Can you work these out from the drawing? Everything is in mm from the part's minimum corner. A direction names the side the tool comes from. Round coordinates to 2 decimals unless told otherwise and drop trailing zeros. Loops run counter-clockwise (first coordinate to the right, second up) from the corner with the lowest first, then second, coordinate; pieces in that order, holes last. Notation, with made-up numbers: (71.25, -27.5) - (129.25, -27.5) arc R22 ccw to (129.25, 11.5) - close; hole circle Ø10 at (42, 18). An arc over 180 degrees is marked (long way). Return JSON: item names as keys, results as strings. Group by question number.
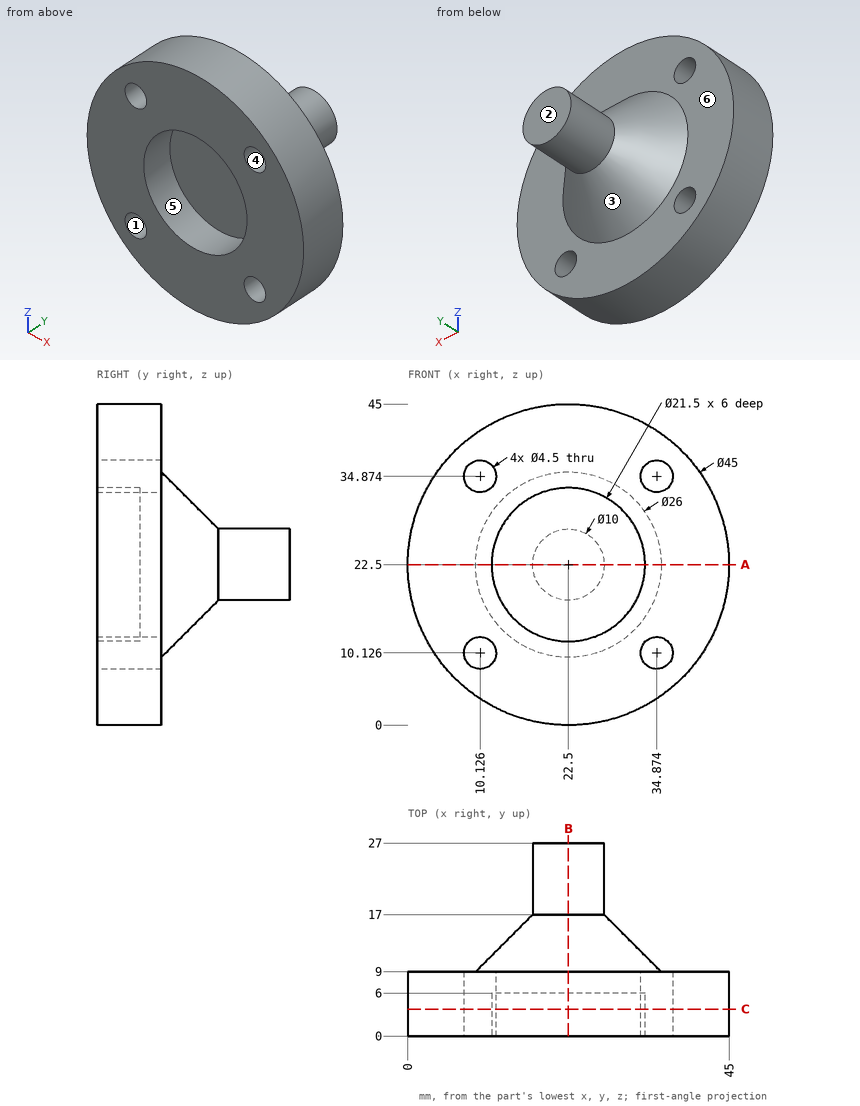
Q1. Imagine slicing it at A-A, the plane z = 22.5. List the corners of the cut face in (x, y) for me, and give its area (3 significant figures).
Q2. Will these pins go through, and if not, where does the flat tip stop? pin 1 Ø12 at (y, z) = (3.5, 39) entering from -X; pin 2 Ø3.5 at (x, z) = (34.87, 34.87) entering from +Y; pin 3 Ø11 at (x, z) = (22, 19.5) entering from -Y; pin 4 Ø5 at (x, z) = (34.87, 10.13) entering from -Y.
Q3. Imagine slicing it at C-C, the plane y = 3.75. Give the number of separate pieces and of enclosed holes in the cut face, and give its area (3 significant figures).
Q4. Imagine slicing it at B-B, the plane x = 22.5. List the corners of the cut face in (y, z) for me.
Q5. If we mould it in two halves opening along X, with no side actions, what happens to the marked faces 1, 2 and 3? For each: +X half, -X half, draft (parallel to the pull), parting line (faces both ways), or undercut.
Q6. For the marked faces 4, 5 and 6, which set-ups out of +Z, -Z, +X, -X, +Y, -Y let a thin tool reach every point of the face, with its end or its side?
Q7. Please list where these lines run through material, in increasing order: line 1 (Z direction, x = 36, y = 7.5) (1 decimal); line 2 (Z direction, x = 22.5, y = 4); line 3 (Z direction, x = 11, y = 1.5).
Output values:
{
 "1": {"outline": "(0, 0) - (11.75, 0) - (11.75, 6) - (33.25, 6) - (33.25, 0) - (45, 0) - (45, 9) - (35.5, 9) - (27.5, 17) - (27.5, 27) - (17.5, 27) - (17.5, 17) - (9.5, 9) - (0, 9) - close", "area": "520 mm^2"},
 "2": {"pin 1": "stops at x = 2.6", "pin 2": "passes through", "pin 3": "stops at y = 6", "pin 4": "stops at y = 0"},
 "3": {"separate pieces": "1", "enclosed holes": "5", "area": "1,160 mm^2"},
 "4": {"outline": "(0, 0) - (9, 0) - (9, 9.5) - (17, 17.5) - (27, 17.5) - (27, 27.5) - (17, 27.5) - (9, 35.5) - (9, 45) - (0, 45) - (0, 33.25) - (6, 33.25) - (6, 11.75) - (0, 11.75) - close"},
 "5": {"face 1": "undercut", "face 2": "draft", "face 3": "parting line"},
 "6": {"face 4": "+Y, -Y", "face 5": "-Y", "face 6": "+Y"},
 "7": {"line 1": "z = 4.5 to 8.2, 12.1 to 32.9, 36.8 to 40.5", "line 2": "z = 0 to 11.75, 33.25 to 45", "line 3": "z = 3.16 to 8.05, 12.2 to 32.8, 36.95 to 41.84"}
}
